Work out the finished part from the listing and answer in its coordinate system (mm). A direction names the side the tool comes from. Coordinates: 2 decimals unless noted, no trailing zeros. Order: outer loops, then holes, each group sorted by start corner. A loop starts at its lowest first (then second) coordinate and runs counter-clockwise, first axis right, second up. Notation, with made-up numbers: (1.5, 68.5) - (10.5, 68.5) arc R27 ccw to (10.5, 101.5) - close; hole circle Ø10 at (-19, -23). An arc over 180 degrees is marked (long way). Answer as a JSON object with one key per item and string values. Group by question number.
1) Find the intervals of material crossed by line 1 along Y through (x, z) = (-0.75, -2.75); line 2 along X through (y, z) = (-1.75, -2); line 3 along Y through (x, z) = (2.5, -2), in increasing order.
2) The mould has two halves that part along Y. Classify faces 4 (the face through (0, 2.25, -3)), 5 (the face through (0, -4, 0)), 6 (the face through (-2, 6, -0.625)): released by +Y, released by -Y, zero draft, split by the parting line, or undercut.
3) Each of these flat-tipped pins is pushed along its axis until it touches: P1, Ø0.7, axis at x = -2.5, y = 2, coming from the +Z side; P2, Ø2, axis at y = 6.5, z = -1.5, coming from the -X side; P3, Ø0.9, axis at x = -1.5, z = 3, coming from the -Y side; P4, Ø1.4, axis at x = 1, z = -1.5, coming from the -Y side. Where does it stop, or does it pass through?
4) Section A-A (y = 0.5) is taken. Give the vertices of the cut face in (x, z) (3 decimals), plus the area to 3 significant figures.
5) Section B-B (z = 0.25) is taken. Give the vertices of the cut face in (x, y), plus the area to 3 significant figures.
6) A tool of negligible diameter and unlimited length cuts with its end or side. For faces 1 (the face through (0, 2.65, -3)), 2 (the face through (2, 6, -0.625)), 3 (the face through (0.05, 1.11, 2.69)), from which of +Z, -Z, +X, -X, +Y, -Y can it reach the whole face along a straight path? Write none if from no direction.
Autodesk Inventor part; units mm, degrees
ref_plane "YZ Plane" through (0, 0, 0) normal (1, 0, 0) x (0, 1, 0)
ref_plane "XZ Plane" through (0, 0, 0) normal (0, 1, 0) x (-1, 0, 0)
ref_plane "XY Plane" through (0, 0, 0) normal (0, 0, 1) x (1, 0, 0)
sketch "Sketch1" plane through (0, 0, 0) normal (0, 1, 0) x (-1, 0, 0)
  line L0 (2.6164, 0.625) -> (1.1164, 0.625)
  line L1 (1.1164, 0.625) -> (1.1164, -0.625)
  line L2 (1.1164, -0.625) -> (2.6164, -0.625)
  line L3 (-2.6164, 0.625) -> (-1.1164, 0.625)
  line L4 (-1.1164, 0.625) -> (-1.1164, -0.625)
  line L5 (-1.1164, -0.625) -> (-2.6164, -0.625)
  line L6 (1.1164, 0) -> (-1.1164, 0) construction
  arc A0 (2.6164, 0.625) -> (-2.6164, 0.625) centre (0, 0) ccw
  arc A1 (-2.6164, -0.625) -> (2.6164, -0.625) centre (0, 0) ccw
  dimension "d1" = 2.69
  dimension "d2" = 2.69
  dimension "d3" = 1.5
  dimension "d4" = 1.25
extrude "Extrusion1" add sketch "Sketch1" along normal blind 2.25
sketch "Sketch2" plane through (0, 2.25, 0) normal (0, 1, 0) x (1, 0, 0)
  line L0 (-1.1164, 0.625) -> (-1.1164, -0.625)
  line L1 (-1.1164, -0.625) -> (-2.6164, -0.625)
  arc A0 (-2.6164, -0.625) -> (2.6164, -0.625) centre (0, 0) ccw construction
  line L2 (2.6164, -0.625) -> (1.1164, -0.625)
  line L3 (1.1164, -0.625) -> (1.1164, 0.625)
  line L4 (1.1164, 0.625) -> (2.6164, 0.625)
  arc A1 (2.6164, 0.625) -> (-2.6164, 0.625) centre (0, 0) ccw construction
  line L5 (-2.6164, 0.625) -> (-1.1164, 0.625)
  arc A2 (-3.4437, -0.625) -> (3.4437, -0.625) centre (0, 0) ccw
  arc A3 (3.4437, 0.625) -> (-3.4437, 0.625) centre (0, 0) ccw
  line L6 (-2.6164, -0.625) -> (-3.4437, -0.625)
  arc A4 (2.6164, 0.625) -> (-2.6164, 0.625) centre (0, 0) ccw construction
  line L7 (-2.6164, 0.625) -> (-3.4437, 0.625)
  line L8 (2.6164, 0.625) -> (3.4437, 0.625)
  line L9 (2.6164, -0.625) -> (3.4437, -0.625)
  dimension "d7" = 3.5
  dimension "d8" = 3.5
extrude "Extrusion2" add sketch "Sketch2" along normal blind 0.4
sketch "Sketch3" plane through (0, 2.65, 0) normal (0, 1, 0) x (1, 0, 0)
  arc A0 (-2.6164, -0.625) -> (2.6164, -0.625) centre (0, 0) ccw
  arc A1 (2.6164, 0.625) -> (-2.6164, 0.625) centre (0, 0) ccw
  line L0 (-3.4437, 0.625) -> (-1.1164, 0.625)
  line L1 (-1.1164, 0.625) -> (-1.1164, -0.625)
  line L2 (-1.1164, -0.625) -> (-3.4437, -0.625)
  line L3 (3.4437, -0.625) -> (1.1164, -0.625)
  line L4 (1.1164, -0.625) -> (1.1164, 0.625)
  line L5 (1.1164, 0.625) -> (3.4437, 0.625)
extrude "Extrusion3" add sketch "Sketch3" along normal blind 13
sketch "Sketch4" plane through (0, 0, 0) normal (0, -1, 0) x (1, 0, 0)
  line L0 (-1.1164, -0.625) -> (-1.1164, 0.625)
  line L1 (-2.6164, -0.625) -> (-1.1164, -0.625)
  arc A0 (-2.6164, -0.625) -> (2.6164, -0.625) centre (0, 0) ccw construction
  line L2 (1.1164, -0.625) -> (2.6164, -0.625)
  line L3 (1.1164, 0.625) -> (1.1164, -0.625)
  line L4 (2.6164, 0.625) -> (1.1164, 0.625)
  arc A1 (2.6164, 0.625) -> (-2.6164, 0.625) centre (0, 0) ccw construction
  line L5 (-1.1164, 0.625) -> (-2.6164, 0.625)
  arc A2 (3.3421, 0.625) -> (-3.3421, 0.625) centre (0, 0) ccw
  arc A3 (-3.3421, -0.625) -> (3.3421, -0.625) centre (0, 0) ccw
  line L6 (2.6164, 0.625) -> (3.3421, 0.625)
  line L7 (3.4437, 0.625) -> (2.6164, 0.625)
  arc A4 (-2.6164, -0.625) -> (2.6164, -0.625) centre (0, 0) ccw
  line L8 (2.6164, -0.625) -> (3.4437, -0.625)
  line L9 (-2.6164, -0.625) -> (-3.3421, -0.625)
  line L10 (-3.4437, -0.625) -> (-2.6164, -0.625)
  line L11 (-2.6164, 0.625) -> (-3.3421, 0.625)
  line L12 (-2.6164, 0.625) -> (-3.4437, 0.625)
  dimension "d13" = 3.4
  dimension "d14" = 3.4
extrude "Extrusion4" add sketch "Sketch4" along normal blind 4
fillet "Fillet1" radius 2 2 edges at (0, 0, -3.4) (0, 0, 3.4)
fillet "Fillet2" radius 2 2 edges at (0, -4, -3.4) (0, -4, 3.4)
equation "\"d2\" = d1"
equation "\"d8\" = d7"
equation "\"d14\" = d13"
properties part number "Toggle_Level" material "PC/ABS Plastic"
Report:
{
 "1": {"line 1": "y = -3.38 to -0.15, 2.25 to 2.65", "line 2": "x = -2.75 to 2.75", "line 3": "y = -2.87 to -0.66, 2.25 to 2.65"},
 "2": {"face 4": "undercut", "face 5": "released by -Y", "face 6": "zero draft"},
 "3": {"P1": "stops at z = 2.68", "P2": "stops at x = -2.62", "P3": "stops at y = -3.32", "P4": "stops at y = -4"},
 "4": {"outline": "(-2.616, -0.625) arc R2.69 ccw to (2.616, -0.625) - (1.116, -0.625) - (1.116, 0.625) - (2.616, 0.625) arc R2.69 ccw to (-2.616, 0.625) - (-1.116, 0.625) - (-1.116, -0.625) - close", "area": "18.9 mm²"},
 "5": {"outline": "(-1.12, -4) - (1.12, -4) - (1.12, 15.65) - (-1.12, 15.65) - close", "area": "43.9 mm²"},
 "6": {"face 1": "-Z, +Y", "face 2": "+X, +Y, -Y", "face 3": "+Z"}
}
